Source: CAD feature listing. Evaluate the final solid. Frame: model axes, mm. Face numbers are marked on the shaded views. A direction names the side the tool comes from. Give positions to 0.01 mm unless a question says otherwise; leave off trailing zeros. Loops run counter-clockwise (first coordinate to the right, second up) from the corner with the lowest first, then second, coordinate; pieces in that order, holes last.
from build123d import *

# Parameters (mm, degrees)
SKIZZE3_W                       = 9
SKIZZE3_H                       = 10.1502367
SKIZZE3_W_2                     = 3.2
SKIZZE3_H_2                     = 6.2
AUFSATZ_LINEAR_AUSTRAGEN2_DEPTH = 4
AUFSATZ_LINEAR_AUSTRAGEN3_DEPTH = 10
SKIZZE6_W                       = 9
SKIZZE6_H                       = 6.8497633
AUFSATZ_LINEAR_AUSTRAGEN5_DEPTH = 4
SKIZZE7_R                       = 1.55688018
SCHNITT_LINEAR_AUSTRAGEN1_DEPTH = 4
SKIZZE8_W                       = 9
SKIZZE8_H                       = 17
SKIZZE8_R                       = 1.55688018
SKIZZE8_W_2                     = 5.098922271
SKIZZE8_H_2                     = 6.2
AUFSATZ_LINEAR_AUSTRAGEN6_DEPTH = 4


with BuildPart() as part:
    # Skizze3 → Aufsatz-Linear austragen2 (new body)
    with BuildSketch(Plane(origin=(0, 0, -22.061362238), x_dir=(-1, 0, 0), z_dir=(0, 0, -1))):
        with Locations((-9.606096766, -3.650507166)):
            Rectangle(SKIZZE3_W, SKIZZE3_H)
        with Locations((-9.155557902, -3.664383383)):
            Rectangle(SKIZZE3_W_2, SKIZZE3_H_2, mode=Mode.SUBTRACT)
    extrude(amount=AUFSATZ_LINEAR_AUSTRAGEN2_DEPTH)

    # Skizze4 → Aufsatz-Linear austragen3 (add)
    with BuildSketch(Plane.XY.offset(-22.061362238)):
        Polygon((12.605305007, 1.424611184), (14.106096766, 1.424611184), (14.106096766, -8.725625516), (12.606096766, -8.725625516), align=None)
    extrude(amount=AUFSATZ_LINEAR_AUSTRAGEN3_DEPTH)

    # Skizze6 → Aufsatz-Linear austragen5 (add)
    with BuildSketch(Plane(origin=(0, 0, -22.061362238), x_dir=(-1, 0, 0), z_dir=(0, 0, -1))):
        with Locations((-9.606096766, 4.849492834)):
            Rectangle(SKIZZE6_W, SKIZZE6_H)
    extrude(amount=AUFSATZ_LINEAR_AUSTRAGEN5_DEPTH)

    # Skizze7 → Schnitt-Linear austragen1 (cut)
    with BuildSketch(Plane(origin=(0, 0, -26.061362238), x_dir=(-1, 0, 0), z_dir=(0, 0, -1))):
        with Locations((-9.606096766, 3.224137783)):
            Circle(SKIZZE7_R)
    extrude(amount=-SCHNITT_LINEAR_AUSTRAGEN1_DEPTH, mode=Mode.SUBTRACT)

    # Skizze8 → Aufsatz-Linear austragen6 (add)
    with BuildSketch(Plane.XY.offset(-12.061362238)):
        with Locations((9.606096766, -0.225625516)):
            Rectangle(SKIZZE8_W, SKIZZE8_H)
        with Locations((9.606096766, 3.224137783)):
            Circle(SKIZZE8_R, mode=Mode.SUBTRACT)
        with Locations((9.155557901, -3.664383383)):
            Rectangle(SKIZZE8_W_2, SKIZZE8_H_2, mode=Mode.SUBTRACT)
    extrude(amount=AUFSATZ_LINEAR_AUSTRAGEN6_DEPTH)


solid = part.part
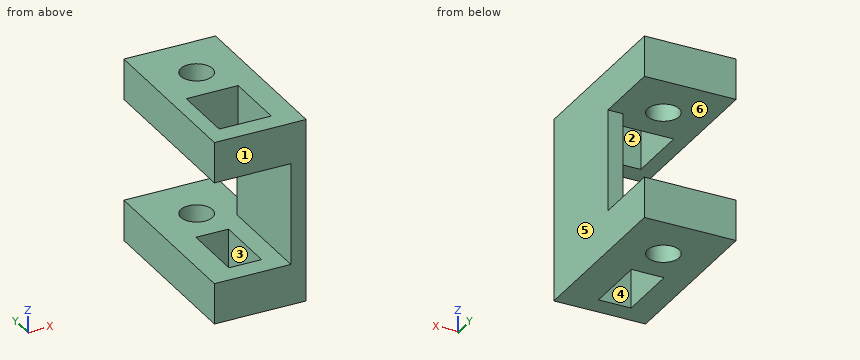
1) Contact query for flat-ended pins moving along their axis: P1, Ø1.5, axis at x = 11.5, z = -15, coming from the -Y side; P2, Ø3, axis at y = -4.5, z = -19, coming from the -X side; P3, Ø4, axis at x = 8, z = -21.5, coming from the +Y side; P4, Ø1.2, axis at x = 13, z = -17, coming from the +Y side. Output: stop coordinate, or through.
Checks:
P1: passes through
P2: stops at x = 12.61
P3: stops at y = 8.27
P4: stops at y = 1.42
2) Cut plane D-D (x = 7). Return loops of the section in (y, z).
Checks:
outline: (-8.73, -26.06) - (8.27, -26.06) - (8.27, -22.06) - (-8.73, -22.06) - close; (-8.73, -12.06) - (-6.76, -12.06) - (-6.76, -8.06) - (-8.73, -8.06) - close; (-0.56, -12.06) - (8.27, -12.06) - (8.27, -8.06) - (-0.56, -8.06) - close
3) Ray query, probe 1 along Z at (x, y) = (8.75, 1); probe 2 along X at (y, z) = (1.25, -21.5); probe 3 along Y at (x, z) = (11.5, -9.5). Return the intervals inside material, ascending.
Checks:
probe 1: z = -26.06 to -22.06, -12.06 to -8.06
probe 2: x = 12.61 to 14.11
probe 3: y = -8.73 to -6.76, -0.56 to 8.27
4) Cut plane C-C (y = -6.25). Return loops of the section in (x, z), and give its area (3 significant figures).
Checks:
outline: (5.11, -26.06) - (7.56, -26.06) - (7.56, -22.06) - (5.11, -22.06) - close; (5.11, -12.06) - (6.61, -12.06) - (6.61, -8.06) - (5.11, -8.06) - close; (10.76, -26.06) - (14.11, -26.06) - (14.11, -8.06) - (11.71, -8.06) - (11.71, -12.06) - (12.61, -12.06) - (12.61, -22.06) - (10.76, -22.06) - close
area: 53.8 mm2
5) Reachability of the marked faces 1, 2 and 3 from +Z, -Z, +X, -X, +Y, -Y: full face, straight path, thin tool, end or side. Return the list, or none.
Checks:
face 1: +Z, -Z, +X, -X, -Y
face 2: +Z
face 3: +Z, -Z
6) Cut plane A-A (x = 6). Return loops of the section in (y, z).
Checks:
outline: (-8.73, -26.06) - (8.27, -26.06) - (8.27, -22.06) - (-8.73, -22.06) - close; (-8.73, -12.06) - (8.27, -12.06) - (8.27, -8.06) - (-8.73, -8.06) - close
7) Cut plane B-B (y = 7.25). Return loops of the section in (x, z).
Checks:
outline: (5.11, -26.06) - (14.11, -26.06) - (14.11, -22.06) - (5.11, -22.06) - close; (5.11, -12.06) - (14.11, -12.06) - (14.11, -8.06) - (5.11, -8.06) - close
8) Pull-direction query (X, two-part tool) for the marked faces 4, 5 and 6; classes: released by +X, released by -X, zero draft, split by the parting line, or undercut.
Checks:
face 4: undercut
face 5: released by +X
face 6: zero draft
